Verification items for the finished model (mm, model axes). A direction names the side the tool comes from. Coordinates: 2 decimals unless noted, no trailing zeros. Loops run counter-clockwise (first coordinate to the right, second up) from the corner with the lowest first, then second, coordinate; pieces in that order, holes last. Notation, with made-up numbers: (-16.75, 88.5) -> (28.25, 88.5) arc R23 ccw to (28.25, 104.5) -> close; hole circle Ø3 at (19, 12). An arc over 180 degrees is marked (long way). Answer as a JSON object with one key per item and string values. Group by question number.
Q1. Set-up check for faces 1 (the flat face through (3.175, 12, -15)), 2 (the flat face through (8, 0, -5)): record each of +Z, -Z, +X, -X, +Y, -Y from which the full face is reachable in a straight line by a thin tool's end or side.
Q2. Cross-section at D-D on z = -10.5. Record the boundary of the cut face in (x, y) (3 decimals).
Q3. Cross-section at A-A on z = -17.78. Record the boundary of the cut face in (x, y) (3 decimals), and give its area (3 significant figures).
Q4. Cross-section at B-B on y = 8.25. Record the boundary of the cut face in (x, z) (3 decimals).
Q5. Release check for a two-part mould opening along X. For faces 3 (the cylindrical face through (4, 10, -6)), 4 (the flat face through (8, 19.05, -5)), 5 (the flat face through (23.65, 9.39, -9.4)) record: released by +X, released by -X, zero draft, split by the parting line, or undercut.
Q6. Scan lines: L1, parallel to Y at x = 2.45, z = -17.78; L2, parallel to X at y = 9.5, z = -8.5 (3 decimals); L3, parallel to X at y = 9, z = -23.75 (3 decimals). Record each from-to range of solid material in increasing order.
Q7. Cross-section at C-C on z = -14. Record the boundary of the cut face in (x, y) (3 decimals), and give its area (3 significant figures).
Q8. Gauge pin test, flat ends, axial feed: pin 1 Ø4 at (x, y) = (21, 16) entering from -Z; pin 2 Ø10 at (x, z) = (9, -14.5) entering from +Y; pin 3 Ø4 at (y, z) = (17, -10.5) entering from +X; pin 4 Ø3 at (x, y) = (10, 12) entering from +Z. Record the tip position at first contact, or that the pin passes through.
```python
from build123d import *

# Parameters (mm, degrees)
BOSS_EXTRUDE1_DEPTH     = 19.05
FILLET1_R               = 2.54
F_1_4_CLEARANCE_HOLE1_D = 6.7564
F_1_4_CLEARANCE_HOLE2_D = 6.7564


with BuildPart() as part:
    # Sketch1 → Boss-Extrude1 (new body)
    with BuildSketch(Plane(origin=(0, 0, 0), x_dir=(1, 0, 0), z_dir=(0, 1, 0))):
        Polygon((0, 0), (0, 25.4), (3.175, 25.4), (3.175, 4.373344438), (23.167823374, 10.885429945), (24.151140547, 7.866537377), align=None)
    extrude(amount=BOSS_EXTRUDE1_DEPTH)

    # Fillet1
    fillet1_edges = [part.edges().sort_by_distance(p)[0] for p in [
        (3.175, 9.525, -4.373344438),
    ]]
    fillet(fillet1_edges, radius=FILLET1_R)

    # 1/4 Clearance Hole1 (through all)
    with Locations(Plane.ZY):
        with Locations((-17.78, 9.525)):
            Hole(F_1_4_CLEARANCE_HOLE1_D / 2)

    # 1/4 Clearance Hole2 (through all)
    with Locations(Plane(origin=(0, 0, 0), x_dir=(0.9508323049826902, 0, -0.30970619593625254), z_dir=(0.30970619593625254, 0, 0.9508323049826902))):
        with Locations((17.78, 9.525)):
            Hole(F_1_4_CLEARANCE_HOLE2_D / 2)


solid = part.part
```
Computed values:
{
 "1": {"face 1": "-Z, +Y, -Y", "face 2": "+Z, -Z, +X, -X, -Y"},
 "2": {"outline": "(0, 0) -> (3.175, 0) -> (3.175, 19.05) -> (0, 19.05) -> close; (21.985, 0) -> (23.293, 0) -> (23.293, 19.05) -> (21.985, 19.05) -> close"},
 "3": {"outline": "(0, 0) -> (3.175, 0) -> (3.175, 6.147) -> (0, 6.147) -> close; (0, 12.903) -> (3.175, 12.903) -> (3.175, 19.05) -> (0, 19.05) -> close", "area": "39.0 mm²"},
 "4": {"outline": "(0, -25.4) -> (3.175, -25.4) -> (3.175, -20.908) -> (0, -20.908) -> close; (0, -14.652) -> (3.175, -14.652) -> (3.175, -7.872) arc R2.54 cw to (6.502, -5.457) -> (12.948, -7.557) -> (13.931, -4.538) -> (0, 0) -> close; (18.897, -9.494) -> (23.168, -10.885) -> (24.151, -7.867) -> (19.88, -6.475) -> close"},
 "5": {"face 3": "undercut", "face 4": "zero draft", "face 5": "released by +X"},
 "6": {"L1": "y = 0 to 6.15, 12.9 to 19.05", "L2": "x = 0 to 3.175, 19.484 to 23.945", "L3": "x = 0 to 3.175"},
 "7": {"outline": "(0, 0) -> (3.175, 0) -> (3.175, 19.05) -> (0, 19.05) -> close", "area": "60.5 mm²"},
 "8": {"pin 1": "stops at z = -10.83", "pin 2": "passes through", "pin 3": "stops at x = 23.94", "pin 4": "stops at z = -2.77"}
}
